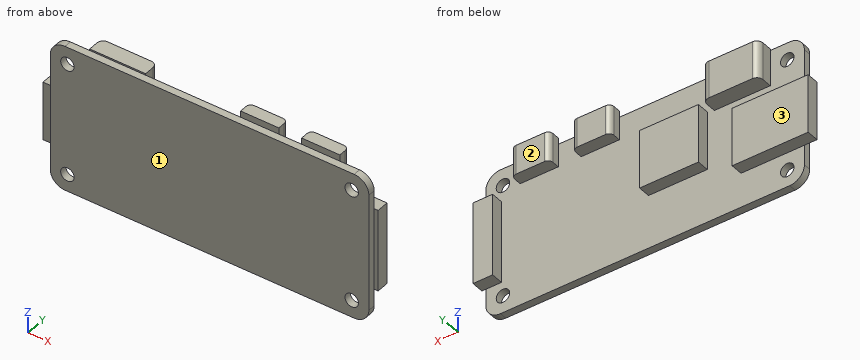
from build123d import *

# Parameters (mm, degrees)
SKETCH_W      = 65
SKETCH_H      = 30
SKETCH_R      = 1.375
PAD_DEPTH     = 1.5
FILLET_R      = 3
SKETCH001_W   = 15.5
SKETCH001_H   = 12
SKETCH001_W_2 = 12
SKETCH001_W_3 = 4
SKETCH001_H_2 = 16.82
SKETCH001_W_4 = 7.8
SKETCH001_H_3 = 6
PAD001_DEPTH  = 2.5
SKETCH002_W   = 11.41
SKETCH002_H   = 7.67
PAD002_DEPTH  = 3.3
FILLET001_R   = 1.25
FILLET002_R   = 1


with BuildPart() as part:
    # Sketch → Pad (new body)
    with BuildSketch(Plane.XZ):
        with Locations((0, 0.07)):
            Rectangle(SKETCH_W, SKETCH_H)
        with Locations((-29, 11.57)):
            Circle(SKETCH_R, mode=Mode.SUBTRACT)
        with Locations((-29, -11.43)):
            Circle(SKETCH_R, mode=Mode.SUBTRACT)
        with Locations((29, -11.43)):
            Circle(SKETCH_R, mode=Mode.SUBTRACT)
        with Locations((29, 11.57)):
            Circle(SKETCH_R, mode=Mode.SUBTRACT)
    extrude(amount=-PAD_DEPTH)

    # Fillet
    fillet_edges = [part.edges().sort_by_distance(p)[0] for p in [
        (-32.5, 0.75, 15.07),
        (-32.5, 0.75, -14.93),
        (32.5, 0.75, -14.93),
        (32.5, 0.75, 15.07),
    ]]
    fillet(fillet_edges, radius=FILLET_R)

    # Sketch001 (on Face5 of Fillet) → Pad001 (join)
    with BuildSketch(Plane(origin=(0, 1.5, 0), x_dir=(1, 0, 0), z_dir=(0, 1, 0))):
        with Locations((-27.32, 1.85)):
            Rectangle(SKETCH001_W, SKETCH001_H)
        with Locations((-6.69, -2.05)):
            Rectangle(SKETCH001_W_2, SKETCH001_H)
        with Locations((31.3, 0.08)):
            Rectangle(SKETCH001_W_3, SKETCH001_H_2)
        with Locations((21.6, -13.37)):
            Rectangle(SKETCH001_W_4, SKETCH001_H_3)
        with Locations((9.15, -13.37)):
            Rectangle(SKETCH001_W_4, SKETCH001_H_3)
    extrude(amount=PAD001_DEPTH)

    # Sketch002 (on Face5 of Pad001) → Pad002 (join)
    with BuildSketch(Plane(origin=(0, 1.5, 0), x_dir=(1, 0, 0), z_dir=(0, 1, 0))):
        with Locations((-19.835, -11.545)):
            Rectangle(SKETCH002_W, SKETCH002_H)
    extrude(amount=PAD002_DEPTH)

    # Fillet001
    fillet001_edges = [part.edges().sort_by_distance(p)[0] for p in [
        (-25.54, 4.8, 11.545),
        (-14.13, 4.8, 11.545),
    ]]
    fillet(fillet001_edges, radius=FILLET001_R)

    # Fillet002
    fillet002_edges = [part.edges().sort_by_distance(p)[0] for p in [
        (5.25, 4, 13.37),
        (13.05, 4, 13.37),
        (17.7, 4, 13.37),
        (25.5, 4, 13.37),
    ]]
    fillet(fillet002_edges, radius=FILLET002_R)


solid = part.part
Design review of the part built by this model. Coordinates are the model's own, in mm. Face numbers are marked on the shaded views. A direction names the side the tool comes from. Round coordinates to 2 decimals unless told otherwise and drop trailing zeros. Order: outer loops, then holes, each group sorted by start corner. A loop starts at its lowest first (then second) coordinate and runs counter-clockwise, first axis right, second up. Notation, with made-up numbers: M -28.75,-16.5 L 17.25,-16.5 A27 cw 17.25,15.5 Z; hole C 50.5,71.25 d10. An arc over 180 degrees is marked long. Answer as CSV lines item,"result". Start each with the question number.
1) Tool access review of the marked faces 1, 2 and 3: name each direction out of +Z, -Z, +X, -X, +Y, -Y from which nothing blocks a thin tool from reaching the whole face with its end or side.
2) Add section A-A (x = -16). Give the boundary of the cut face in (y, z), then the cut area to 3 significant figures.
3) Add section D-D (z = 0). Give the boundary of the cut face in (x, y).
4) Add section C-C (x = 23). Give the boundary of the cut face in (y, z), then the cut area to 3 significant figures.
5) Wall thickness on line 1 along Z through (x, y) = (29, 0.5) (3 decimals); line 2 along X through (y, z) = (1.6, -5.5); line 3 along Y through (x, z) = (-0.5, 10): over which ranges is each line inside the solid? List them lowest first. Write a range as [from, to].
6) For pin 1 Ø6.5 at (x, z) = (8, 14) entering from +Y; pin 2 Ø1.6 at (y, z) = (2.5, 14) entering from -X; pin 3 Ø1.6 at (x, y) = (-20, 3) entering from -Z, all flat-tipped, find the tip position at first contact; note any pin that passes through.
7) Add section B-B (z = 7). Give the boundary of the cut face in (x, y), then the cut area to 4 significant figures.
Resolved:
1,face 1,"+Z, -Z, +X, -X, -Y"
1,face 2,"+Z, -Z, +X, +Y"
1,face 3,"-Z, +X, -X, +Y"
2,outline,"M 0,-14.93 L 1.5,-14.93 L 1.5,7.71 L 4.8,7.71 L 4.8,15.38 L 1.5,15.38 L 1.5,15.07 L 0,15.07 Z"
2,area,"70.3 mm^2"
3,outline,"M -35.07,1.5 L -32.5,1.5 L -32.5,0 L 32.5,0 L 32.5,1.5 L 33.3,1.5 L 33.3,4 L 29.3,4 L 29.3,1.5 L -0.69,1.5 L -0.69,4 L -12.69,4 L -12.69,1.5 L -19.57,1.5 L -19.57,4 L -35.07,4 Z"
4,outline,"M 0,-14.93 L 1.5,-14.93 L 1.5,10.37 L 4,10.37 L 4,16.37 L 1.5,16.37 L 1.5,15.07 L 0,15.07 Z"
4,area,"60.0 mm^2"
5,line 1,"[-14.93, -12.805], [-10.055, 10.195], [12.945, 15.07]"
5,line 2,"[-35.07, -19.57], [29.3, 33.3]"
5,line 3,"[0, 1.5]"
6,pin 1,"y = 4"
6,pin 2,"x = -25.54"
6,pin 3,"z = -7.85"
7,outline,"M -32.5,0 L 32.5,0 L 32.5,1.5 L 33.3,1.5 L 33.3,4 L 29.3,4 L 29.3,1.5 L -0.69,1.5 L -0.69,4 L -12.69,4 L -12.69,1.5 L -32.5,1.5 Z"
7,area,"137.5 mm^2"
